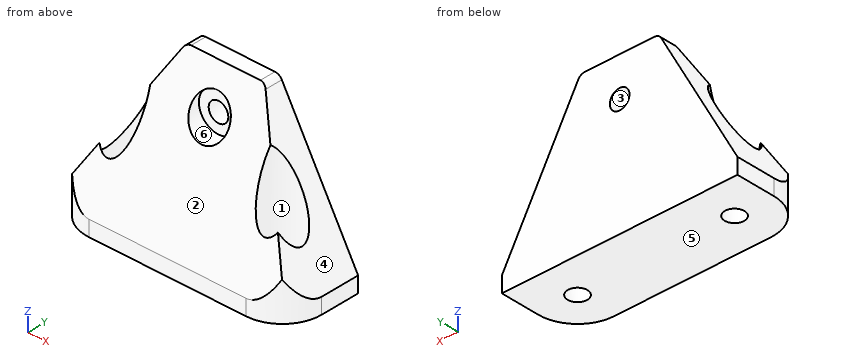
from build123d import *

# Parameters (mm, degrees)
SKETCH_W         = 60
SKETCH_H         = 20
PAD_DEPTH        = 40
POCKET_DEPTH     = 20.001
HOLE_D           = 5
HOLE_DEPTH       = 25
HOLE_CBORE_D     = 10
HOLE_CBORE_DEPTH = 14
POCKET001_DEPTH  = 60.001
SKETCH004_R      = 5
HOLE001_DEPTH    = 36
SKETCH005_R      = 2.5
POCKET002_DEPTH  = 5
FILLET_R         = 10
FILLET001_R      = 2


with BuildPart() as part:
    # Sketch → Pad (new body)
    with BuildSketch(Plane.XY):
        Rectangle(SKETCH_W, SKETCH_H)
    extrude(amount=PAD_DEPTH)

    # Sketch001 (on Face3 of Pad) → Pocket (cut, through all)
    with BuildSketch(Plane.XZ.offset(10)):
        Polygon((30, 40), (30, 4), (10, 40), align=None)
        Polygon((-30, 4), (-30, 40), (-10, 40), align=None)
    extrude(amount=-POCKET_DEPTH, mode=Mode.SUBTRACT)

    # Hole
    with Locations(Plane.XZ.offset(10)):
        with Locations((0, 30)):
            CounterBoreHole(HOLE_D / 2, HOLE_CBORE_D / 2, HOLE_CBORE_DEPTH, depth=HOLE_DEPTH)

    # Sketch003 (on Face4 of Hole) → Pocket001 (cut, through all)
    with BuildSketch(Plane.YZ.offset(30)):
        Polygon((-10, 4), (-10, 40), (6, 40), align=None)
    extrude(amount=-POCKET001_DEPTH, mode=Mode.SUBTRACT)

    # Sketch004 (on Face7 of Pocket001) → Hole001 (cut)
    with BuildSketch(Plane.XY.offset(40)):
        with Locations((-20, 0)):
            Circle(SKETCH004_R)
        with Locations((20, 0)):
            Circle(SKETCH004_R)
    extrude(amount=-HOLE001_DEPTH, mode=Mode.SUBTRACT)

    # Sketch005 (on Face15 of Hole001) → Pocket002 (cut)
    with BuildSketch(Plane.XY.offset(4)):
        with Locations((-20, 0)):
            Circle(SKETCH005_R)
        with Locations((20, 0)):
            Circle(SKETCH005_R)
    extrude(amount=-POCKET002_DEPTH, mode=Mode.SUBTRACT)

    # Fillet
    fillet_edges = [part.edges().sort_by_distance(p)[0] for p in [
        (30, -10, 2),
        (-30, -10, 2),
    ]]
    fillet(fillet_edges, radius=FILLET_R)

    # Fillet001
    fillet001_edges = [part.edges().sort_by_distance(p)[0] for p in [
        (10, 8, 40),
        (-10, 8, 40),
    ]]
    fillet(fillet001_edges, radius=FILLET001_R)


solid = part.part
Part model, mm, in its own coordinate system. Face numbers are marked on the shaded views. A direction names the side the tool comes from. Round coordinates to 2 decimals unless told otherwise and drop trailing zeros. Loops run counter-clockwise (first coordinate to the right, second up) from the corner with the lowest first, then second, coordinate; pieces in that order, holes last. Notation, with made-up numbers: (65, 28) - (108, 28) arc R7 ccw to (108, 33) - close; hole circle Ø5 at (-34.5, -39.75). An arc over 180 degrees is marked (long way). Answer as a JSON object with one key per item and string values.
Item 1: Band-saw the part on C-C on z = 19.5. List the corners of the cut face in (x, y).
Output:
{"outline": "(-21.39, 4.8) arc R5 cw to (-16.09, -3.11) - (16.09, -3.11) arc R5 cw to (21.39, 4.8) - (21.39, 10) - (-21.39, 10) - close"}
Item 2: Band-saw the part on B-B on x = 1.5. List the corners of the cut face in (y, z), plus the area to 3 significant figures.
Output:
{"outline": "(-10, 0) - (10, 0) - (10, 28) - (4, 28) - (4, 25.23) - (-0.56, 25.23) - (-10, 4) - close; (3.68, 34.77) - (4, 34.77) - (4, 32) - (10, 32) - (10, 40) - (6, 40) - close", "area": "465 mm2"}
Item 3: Pull direction Z, two halves, no side cores. Call the marked faces 3, 4, 5 and 6: pulls with the +Z half, pulls with the -Z half, needs draft (parallel to the pull), parting line crosses it, or undercut.
Output:
{"face 3": "undercut", "face 4": "pulls with the +Z half", "face 5": "pulls with the -Z half", "face 6": "undercut"}
Item 4: Band-saw the part on A-A on z = 3. List the corners of the cut face in (x, y), plus the area to 3 significant figures.
Output:
{"outline": "(-30, 0) arc R10 ccw to (-20, -10) - (20, -10) arc R10 ccw to (30, 0) - (30, 10) - (-30, 10) - close; hole circle Ø5 at (-20, 0); hole circle Ø5 at (20, 0)", "area": "1,120 mm2"}
Item 5: Tool access for the marked faces 1 and 2: list every direction of +Z, -Z, +X, -X, +Y, -Y with a clear straight run to the whole face (end or side of a thin tool).
Output:
{"face 1": "+Z", "face 2": "+Z, +X, -X, -Y"}
Item 6: Pin check, flat tips, straight feed: pin 1 (4.5 mm diameter, centred on x = 20, y = 0, fed in from -Z); pin 2 (1.5 mm diameter, centred on x = -17, y = 0.5, fed in from +Z); pin 3 (4 mm diameter, centred on x = -16.5, z = 31, fed in from -Y); pin 4 (6 mm diameter, centred on x = 0, z = 30, fed in from -Y). Stop position of each tip, or through.
Output:
{"pin 1": "through", "pin 2": "z = 4", "pin 3": "y = 1.33", "pin 4": "y = 4"}
Item 7: Wall check: L1, parallel to Y at x = 20, z = 1.55; L2, parallel to Y at x = -20, z = 21; L3, parallel to X at y = 4.5, z = 8.5. Give the ranges that are in metal, low to high.
Output:
{"L1": "-10 to -2.5, 2.5 to 10", "L2": "5 to 10", "L3": "-27.5 to -22.18, -17.82 to 17.82, 22.18 to 27.5"}
